from build123d import *

# Parameters (mm, degrees)
SKETCH1_W                = 54
SKETCH1_H                = 60
BOSS_EXTRUDE1_DEPTH      = 4
BOSS_EXTRUDE2_DEPTH      = 6
BOSS_EXTRUDE2_DEPTH_BACK = 60
SKETCH2_W                = 10
SKETCH2_H                = 17
SKETCH3_W                = 28
SKETCH3_H                = 13
BOSS_EXTRUDE3_DEPTH      = 66
SKETCH9_W                = 56
SKETCH9_H                = 28
CUT_EXTRUDE3_DEPTH       = 13
SKETCH10_W               = 5
SKETCH10_H               = 28
BOSS_EXTRUDE6_DEPTH      = 4
SKETCH11_R               = 2.25
CUT_EXTRUDE5_DEPTH       = 91.138781887
SKETCH12_W               = 5
SKETCH12_H               = 17
BOSS_EXTRUDE7_DEPTH      = 4
CUT_EXTRUDE6_DEPTH       = 91.138781887
FILLET3_R                = 1
BOSS_EXTRUDE8_DEPTH      = 10
BOSS_EXTRUDE8_DEPTH_BACK = 5
SKETCH14_R               = 4
SKETCH15_W               = 17
SKETCH15_H               = 8
BOSS_EXTRUDE9_DEPTH      = 5
SKETCH16_R               = 6
BOSS_EXTRUDE11_DEPTH     = 12
SKETCH17_R               = 6
CUT_EXTRUDE7_DEPTH       = 5
CHAMFER1_SIZE            = 9.326153163
CHAMFER1_SIZE_2          = 20
SKETCH18_W               = 66
SKETCH18_H               = 5
BOSS_EXTRUDE14_DEPTH     = 17
FILLET8_R                = 15
FILLET9_R                = 15


with BuildPart() as part:
    # Sketch1 → Boss-Extrude1 (new body)
    with BuildSketch(Plane(origin=(0, 0, 0), x_dir=(1, 0, 0), z_dir=(0, 1, 0))):
        with Locations((27, 30)):
            Rectangle(SKETCH1_W, SKETCH1_H)
    extrude(amount=BOSS_EXTRUDE1_DEPTH)

    # Sketch2 → Boss-Extrude2 (add, two sides: drawn at the far end of the back side and taken through both)
    with BuildSketch(Plane(origin=(54, 0, 0), x_dir=(0, 0, -1), z_dir=(1, 0, 0)).offset(-BOSS_EXTRUDE2_DEPTH_BACK)):
        with Locations((5, -4.5)):
            Rectangle(SKETCH2_W, SKETCH2_H)
    extrude(amount=BOSS_EXTRUDE2_DEPTH + BOSS_EXTRUDE2_DEPTH_BACK)

    # Sketch3 → Boss-Extrude3 (add, through all)
    with BuildSketch(Plane(origin=(60, 0, 0), x_dir=(0, 0, -1), z_dir=(1, 0, 0))):
        with Locations((-14, -6.5)):
            Rectangle(SKETCH3_W, SKETCH3_H)
    extrude(amount=-BOSS_EXTRUDE3_DEPTH)

    # Sketch9 → Cut-Extrude3 (cut)
    with BuildSketch(Plane(origin=(0, 0, 0), x_dir=(1, 0, 0), z_dir=(0, 1, 0))):
        with Locations((27, -14)):
            Rectangle(SKETCH9_W, SKETCH9_H)
    extrude(amount=-CUT_EXTRUDE3_DEPTH, mode=Mode.SUBTRACT)

    # Sketch10 → Boss-Extrude6 (add)
    with BuildSketch(Plane(origin=(0, 0, 0), x_dir=(1, 0, 0), z_dir=(0, 1, 0))):
        with Locations((-3.5, -14)):
            Rectangle(SKETCH10_W, SKETCH10_H)
        with Locations((57.5, -14)):
            Rectangle(SKETCH10_W, SKETCH10_H)
    extrude(amount=BOSS_EXTRUDE6_DEPTH)

    # Sketch11 → Cut-Extrude5 (cut, through all)
    with BuildSketch(Plane(origin=(60, 0, 0), x_dir=(0, 0, -1), z_dir=(1, 0, 0))):
        with BuildLine():
            Line((-22.048344565, -2.614854966), (-23, -2.5))
            ThreePointArc((-23, -2.5), (-27, -6.5), (-23, -10.5))
            Line((-23, -10.5), (-22.048344565, -10.385145034))
            ThreePointArc((-22.048344565, -10.385145034), (-19.853047368, -8.96914745), (-19, -6.5))
            ThreePointArc((-19, -6.5), (-19.853047368, -4.03085255), (-22.048344565, -2.614854966))
        make_face()
        with BuildLine():
            Line((-8.5, -4.25), (-22.048344565, -2.614854966))
            ThreePointArc((-22.048344565, -2.614854966), (-19.853047368, -4.03085255), (-19, -6.5))
            ThreePointArc((-19, -6.5), (-19.853047368, -8.96914745), (-22.048344565, -10.385145034))
            Line((-22.048344565, -10.385145034), (-8.5, -8.75))
            ThreePointArc((-8.5, -8.75), (-10.75, -6.5), (-8.5, -4.25))
        make_face()
        with Locations((-8.5, -6.5)):
            Circle(SKETCH11_R)
    extrude(amount=-CUT_EXTRUDE5_DEPTH, mode=Mode.SUBTRACT)

    # Sketch12 → Boss-Extrude7 (add)
    with BuildSketch(Plane.XY.offset(28)):
        with Locations((57.5, -4.5)):
            Rectangle(SKETCH12_W, SKETCH12_H)
        with Locations((-3.5, -4.5)):
            Rectangle(SKETCH12_W, SKETCH12_H)
    extrude(amount=BOSS_EXTRUDE7_DEPTH)

    # Sketch13 → Cut-Extrude6 (cut, through all)
    with BuildSketch(Plane.ZY.offset(6)):
        with BuildLine():
            Line((29.5, -6.5), (29.5, 4))
            Line((29.5, 4), (32, 4))
            Line((32, 4), (32, -13))
            Line((32, -13), (23, -13))
            ThreePointArc((23, -13), (27.596194078, -11.096194078), (29.5, -6.5))
        make_face()
    extrude(amount=-CUT_EXTRUDE6_DEPTH, mode=Mode.SUBTRACT)

    # Fillet3
    fillet3_edges = [part.edges().sort_by_distance(p)[0] for p in [
        (27, 0, -60),
    ]]
    fillet(fillet3_edges, radius=FILLET3_R)

    # Sketch14 → Boss-Extrude8 (add, two sides: drawn at the far end of the back side and taken through both)
    with BuildSketch(Plane(origin=(-1, 0, 0), x_dir=(0, 0, -1), z_dir=(1, 0, 0)).offset(-BOSS_EXTRUDE8_DEPTH_BACK)):
        with Locations((-23, -6.5)):
            Circle(SKETCH14_R)
    extrude(amount=BOSS_EXTRUDE8_DEPTH + BOSS_EXTRUDE8_DEPTH_BACK)

    # Sketch15 → Boss-Extrude9 (add)
    with BuildSketch(Plane(origin=(-1, 0, 0), x_dir=(0, 0, -1), z_dir=(1, 0, 0))):
        with Locations((-14.5, -6.5)):
            Rectangle(SKETCH15_W, SKETCH15_H)
    extrude(amount=-BOSS_EXTRUDE9_DEPTH)

    # Sketch16 → Boss-Extrude11 (add)
    with BuildSketch(Plane(origin=(9, 0, 0), x_dir=(0, 0, -1), z_dir=(1, 0, 0))):
        with Locations((-23, -6.5)):
            Circle(SKETCH16_R)
    extrude(amount=-BOSS_EXTRUDE11_DEPTH)

    # Sketch17 → Cut-Extrude7 (cut)
    with BuildSketch(Plane(origin=(9, 0, 0), x_dir=(0, 0, -1), z_dir=(1, 0, 0))):
        with Locations((-23, -6.5)):
            Circle(SKETCH17_R)
    extrude(amount=-CUT_EXTRUDE7_DEPTH, mode=Mode.SUBTRACT)

    # Chamfer1
    # the kernel refuses this chamfer: 20, 9.326153163 mm, written as the material it takes off along each edge
    with BuildSketch(Plane(origin=(55, 4, 0), x_dir=(0, 0.07481330637059955, -0.9971975577536774), z_dir=(-1, 0, 0))) as chamfer1_piece_1:
        Polygon((CHAMFER1_SIZE * 0.997197557764, CHAMFER1_SIZE * 0.0748133063714), (-CHAMFER1_SIZE_2 * 0.0748133063706, CHAMFER1_SIZE_2 * 0.997197557754), (0, 0), align=None)
    extrude(amount=56, mode=Mode.SUBTRACT)

    # Sketch18 → Boss-Extrude14 (add)
    with BuildSketch(Plane(origin=(0, 4, 0), x_dir=(1, 0, 0), z_dir=(0, 1, 0))):
        with Locations((27, 12.5)):
            Rectangle(SKETCH18_W, SKETCH18_H)
    extrude(amount=-BOSS_EXTRUDE14_DEPTH)

    # Fillet8
    # the kernel refuses this fillet: 15 mm, written as the material it adds along each edge
    with BuildSketch(Plane(origin=(54, 0, -15), x_dir=(0, -1, 0), z_dir=(-1, 0, 0))) as fillet8_piece_1:
        with BuildLine():
            CenterArc((15, -14.866068747), FILLET8_R, 97.662255661, 82.337744339)
            Line((0, -14.866068747), (-0.3, -14.866068747))
            Line((-0.3, -14.866068747), (-0.3, 0))
            Line((-0.3, 0), (0, 0.3))
            ThreePointArc((0, 0.3), (6.5, 0.3), (12.96, 0.297321375))
            Line((12.96, 0.297321375), (13, 0))
        make_face()
    extrude(amount=54)

    # Fillet9
    # the kernel refuses this fillet: 15 mm, written as the material it adds along each edge
    with BuildSketch(Plane(origin=(54, 4, -15), x_dir=(1, 0, 0), z_dir=(0, -1, 0))) as fillet9_piece_1_section:
        with BuildLine():
            CenterArc((15, -12), FILLET9_R, 126.869897646, 53.130102354)
            Line((0, -12), (0, 0))
            Line((0, 0), (6, 0))
        make_face()
    fillet9_piece_1 = extrude(amount=17, mode=Mode.PRIVATE)
    fillet9_piece_1 = fillet9_piece_1 - Plane(origin=(58.238574597, -15, -29.866068747), x_dir=(0, -1, 0), z_dir=(1, 0, 0)) * Cylinder(15, 83, mode=Mode.PRIVATE)
    add(fillet9_piece_1)
    with BuildSketch(Plane(origin=(0, -13, -15), x_dir=(0, 0, -1), z_dir=(0, 1, 0))) as fillet9_piece_2_section:
        with BuildLine():
            CenterArc((12, 15), FILLET9_R, 216.869897646, 53.130102354)
            Line((0, 6), (0, 0))
            Line((0, 0), (12, 0))
        make_face()
    fillet9_piece_2 = extrude(amount=17, mode=Mode.PRIVATE)
    fillet9_piece_2 = fillet9_piece_2 - Plane(origin=(-0.149142202, -15, -29.866068747), x_dir=(0, -1, 0), z_dir=(1, 0, 0)) * Cylinder(15, 82, mode=Mode.PRIVATE)
    add(fillet9_piece_2)


solid = part.part
Geometry: final body of the model. Coordinates: model frame, mm. A direction names the side the tool comes from. Round coordinates to 2 decimals unless told otherwise and drop trailing zeros. Loops run counter-clockwise (first coordinate to the right, second up) from the corner with the lowest first, then second, coordinate; pieces in that order, holes last. Notation, with made-up numbers: M -38,89.25 L -14,89.25 A11 ccw -14,99.25 Z; hole C 74,58.25 d5. An arc over 180 degrees is marked long. Put each result on its own line as item: value. Start each with the question number.
(1) Set-up query: faces 1 (the face through (57.54, -6.55, 6.25)), 2 (the face through (-4, -1, 29.5)), 3 (the face through (0, 2, -43)), 4 (the face through (27, 4, -26)), 5 (the face through (27, 0, -45)). Return all of +Z, -Z, +X, -X, +Y, -Y with unobstructed straight access to the full face (end or side cutting, diameter ignored); none if empty.
(2) Section query C-C (x = 56). Return loops of the section in (y, z).
(3) Material intervals for line 1 along X through (y, z) = (-8.5, 20); line 2 along X through (y, z) = (1, 6); line 3 along Y through (x, z) = (53, -33), sorted ascending. Write a range as [from, to].
(4) Contact query for flat-ended pins moving along their axis: pin 1 Ø3 at (x, y) = (33.5, 0.5) entering from -Z; pin 2 Ø1.5 at (x, y) = (32, -2.5) entering from +Z; pin 3 Ø2 at (y, z) = (2.5, -41.5) entering from -X; pin 4 Ø4.5 at (y, z) = (1, -47.5) entering from +X. Output: stop coordinate, or through.
(5) Draft query along X for faces 6 (the face through (55, -2, 10)), 7 (the face through (27, 2, -60)), 8 (the face through (-6, -4, 8)), 9 (the face through (54, 2, -43)). Return one class per face: +X half, -X half, draft (parallel to the pull), parting line (faces both ways), or undercut.
(6) Section query D-D (y = 2.25). Return loops of the section in (x, z).
(7) Section query B-B (y = -5.5). Return loops of the section in (x, z), then the cut area to 3 significant figures.
(8) Section query A-A (x = 44.5). Return loops of the section in (y, z).
Findings below:
1. face 1: +X
1. face 2: +Z, +X, -X, +Y, -Y
1. face 3: -Z, -X, +Y, -Y
1. face 4: +Z, -Z, +X, -X, +Y
1. face 5: -Z, +X, -X, -Y
2. outline: M -13,-15 A15 cw -4.14,-19.52 L 4,-19.52 L 4,29.5 L -6.5,29.5 A6.5 ccw -13,23 Z; hole M -10.5,23 L -8.75,8.5 A2.25 ccw -4.25,8.5 L -2.5,23 A4 ccw Z
3. line 1: x = [-6, 4]
3. line 2: x = [-6, -1], [55, 60]
3. line 3: y = [0, 4]
4. pin 1: stops at z = -60
4. pin 2: stops at z = -5.95
4. pin 3: stops at x = 0
4. pin 4: stops at x = 54
5. face 6: undercut
5. face 7: draft
5. face 8: -X half
5. face 9: +X half
6. outline: M -6,-15 A15 cw 0,-27 L 0,-60 L 54,-60 L 54,-27 A15 cw 60,-15 L 60,29.5 L 55,29.5 L 55,-8.51 L -1,-8.51 L -1,29.5 L -6,29.5 Z
7. outline: M -6,-15 A15 cw -2.81,-18.26 L 56.81,-18.26 A15 cw 60,-15 L 60,6.48 L 55,6.48 L 55,-4.9 L -1,-4.9 L -1,17.08 L 4,17.08 L 4,28.92 L -1,28.92 L -1,29.5 L -6,29.5 Z; M 55,26.87 L 60,26.87 L 60,29.5 L 55,29.5 Z
7. area: 1,170 mm2
8. outline: M -13,-15 A15 cw 0,-29.87 L 0,-59 A1 ccw 1,-60 L 4,-60 L 4,-9.33 L -13,-1.4 Z
